Work out the finished part from the listing and answer in its coordinate system (mm). A direction names the side the tool comes from. Round coordinates to 2 decimals unless told otherwise and drop trailing zeros. Loops run counter-clockwise (first coordinate to the right, second up) from the corner with the lowest first, then second, coordinate; pieces in that order, holes last. Notation, with made-up numbers: (-30, 39) -> (19, 39) arc R8 cw to (19, 47) -> close; hole circle Ø11 at (76.25, -16.75). An arc over 180 degrees is marked (long way). Use one line per item in the form item = value.
```python
from build123d import *

# Parameters (mm, degrees)
SKETCH1_R           = 9
BOSS_EXTRUDE1_DEPTH = 16.4
SKETCH2_W           = 6
SKETCH2_H           = 13
FILLET1_R           = 5
FILLET2_R           = 1


with BuildPart() as part:
    # Sketch1 → Boss-Extrude1 (new body)
    with BuildSketch(Plane(origin=(0, 0, 0), x_dir=(1, 0, 0), z_dir=(0, 1, 0))):
        with Locations(Location((0, 0, 0), (0, 0, 270))):
            Circle(SKETCH1_R)
    extrude(amount=BOSS_EXTRUDE1_DEPTH)

    # Sketch2 → Ø12.0mm Dowel Hole1 (revolve, cut)
    with BuildSketch(Plane(origin=(0, 16.4, 0), x_dir=(0, 0, 1), z_dir=(1, 0, 0))):
        with Locations((3, 6.5)):
            Rectangle(SKETCH2_W, SKETCH2_H)
    revolve(axis=Axis((0, 19.332571692, 0), (0, -1, 0)), mode=Mode.SUBTRACT)

    # Sketch3 → Cut-Revolve1 (revolve, cut)
    with BuildSketch(Plane(origin=(0, 0, 0), x_dir=(0, 0, -1), z_dir=(1, 0, 0))):
        Polygon((-9, 0), (-1.686427948, 0), (-9, 4.39443743), align=None)
    revolve(axis=Axis((0, 0, 0), (0, 1, 0)), mode=Mode.SUBTRACT)

    # Fillet1
    fillet1_edges = [part.edges().sort_by_distance(p)[0] for p in [
        (0, 3.4, -6),
    ]]
    fillet(fillet1_edges, radius=FILLET1_R)

    # Fillet2
    fillet2_edges = [part.edges().sort_by_distance(p)[0] for p in [
        (0, 16.4, -6),
    ]]
    fillet(fillet2_edges, radius=FILLET2_R)


solid = part.part
```
(1) Find section A-A, the plane y = 9.25. Write down the section's boundary in (x, z), then the cut area to 3 significant figures.
Completed:
outline = circle Ø18 at (0, 0); hole circle Ø12 at (0, 0)
area = 141 mm2
(2) Consider L1, parallel to X at y = 12.25, z = 0; L2, parallel to X at y = 10.5, z = -5.5; L3, parallel to Z at x = -2.5, y = 9.25. Determine where each line is inside the solid, lowest interval first.
Completed:
L1 = -9 to -6, 6 to 9
L2 = -7.12 to -2.4, 2.4 to 7.12
L3 = -8.65 to -5.45, 5.45 to 8.65
(3) For faces 4 (the conical face through (-1.305, 0.275, -1.701)), 5 (the flat face through (0, 3.4, 0)), determine the directions among +Z, -Z, +X, -X, +Y, -Y from which every point of the face is accessible in a straight line to the end or side of a thin tool.
Completed:
face_4 = -Y
face_5 = +Y
(4) Given P1, Ø1, axis at x = -7, z = -4, coming from the -Y side; P2, Ø0.6, axis at x = 0, z = 0, coming from the +Y side; P3, Ø1, axis at x = 2, y = 12.5, coming from the -Z side; P4, Ø5, axis at y = 10.5, z = 2, coming from the -X side, each flat-ended and moving along its own axis, determine where each tip first touches the part or whether it passes through.
Completed:
P1 = 3.53
P2 = 3.4
P3 = -8.87
P4 = -9
(5) For a pull along X with two mould halves and no side action, classify faces 1 (the cylindrical face through (2.703, 10.313, 8.584)), 2 (the flat face through (0, 0, 0)), 3 (the cylindrical face through (0, 12, -6)) as +X half, -X half, draft (parallel to the pull), parting line (faces both ways), or undercut.
Completed:
face_1 = parting line
face_2 = draft
face_3 = undercut
